The listing builds one solid part. Answer for the finished solid, in the listing's coordinates (mm). Round coordinates to 2 decimals unless told otherwise and drop trailing zeros. Order: outer loops, then holes, each group sorted by start corner. A loop starts at its lowest first (then second) coordinate and runs counter-clockwise, first axis right, second up. Notation, with made-up numbers: (13.25, 79) -> (50.25, 79) arc R30 cw to (50.25, 110) -> close; hole circle Ø6 at (-16, 64). An arc over 180 degrees is marked (long way). Answer in a Markdown table with one row per item. Add a question column.
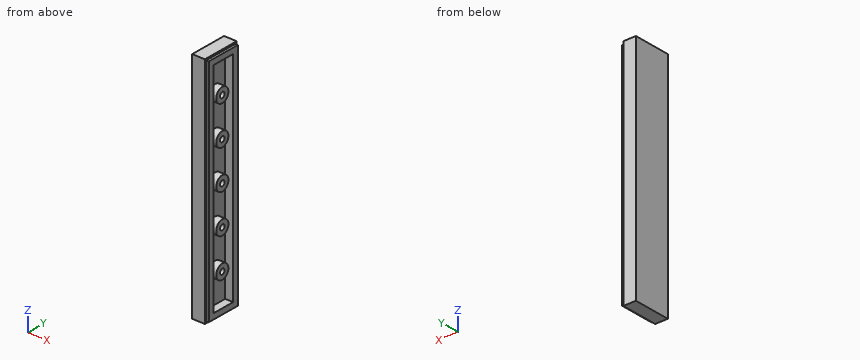
```python
from build123d import *

# Parameters (mm, degrees)
SKETCH1_W           = 47.79
SKETCH1_H           = 7.79
BOSS_EXTRUDE1_DEPTH = 2.63
SHELL1_T            = -1.5
SKETCH2_W           = 47.09
SKETCH2_H           = 7.09
SKETCH2_W_2         = 44.79
SKETCH2_H_2         = 4.79
BOSS_EXTRUDE2_DEPTH = 0.52
SKETCH3_R           = 1.485
SKETCH3_R_2         = 0.555
BOSS_EXTRUDE3_DEPTH = 1.45


with BuildPart() as part:
    # Sketch1 → Boss-Extrude1 (new body)
    with BuildSketch(Plane(origin=(0, 0, 0), x_dir=(0, 0, -1), z_dir=(1, 0, 0))):
        Rectangle(SKETCH1_W, SKETCH1_H)
    extrude(amount=BOSS_EXTRUDE1_DEPTH)

    # Shell1
    shell1_openings = [part.faces().sort_by_distance(p)[0] for p in [
        (2.63, 0, 0),
    ]]
    offset(amount=SHELL1_T, openings=shell1_openings, kind=Kind.INTERSECTION)

    # Sketch2 → Boss-Extrude2 (add)
    with BuildSketch(Plane(origin=(2.63, 0, 0), x_dir=(0, 0, -1), z_dir=(1, 0, 0))):
        Rectangle(SKETCH2_W, SKETCH2_H)
        Rectangle(SKETCH2_W_2, SKETCH2_H_2, mode=Mode.SUBTRACT)
    extrude(amount=BOSS_EXTRUDE2_DEPTH)

    # Sketch3 → Boss-Extrude3 (add)
    # profile 1 of 5: a face of its own
    with BuildSketch(Plane(origin=(1.5, 0, 0), x_dir=(0, 0, -1), z_dir=(1, 0, 0))):
        with Locations(Location((-15.93, 0, 0), (0, 0, 180))):
            Circle(SKETCH3_R)
        with Locations(Location((-15.93, 0, 0), (0, 0, 180))):
            Circle(SKETCH3_R_2, mode=Mode.SUBTRACT)
    # profile 2 of 5: a face of its own
    with BuildSketch(Plane(origin=(1.5, 0, 0), x_dir=(0, 0, -1), z_dir=(1, 0, 0))):
        with Locations(Location((-7.96, 0, 0), (0, 0, 180))):
            Circle(SKETCH3_R)
        with Locations(Location((-7.96, 0, 0), (0, 0, 180))):
            Circle(SKETCH3_R_2, mode=Mode.SUBTRACT)
    # profile 3 of 5: a face of its own
    with BuildSketch(Plane(origin=(1.5, 0, 0), x_dir=(0, 0, -1), z_dir=(1, 0, 0))):
        with Locations(Location((0.01, 0, 0), (0, 0, 180))):
            Circle(SKETCH3_R)
        with Locations(Location((0.01, 0, 0), (0, 0, 180))):
            Circle(SKETCH3_R_2, mode=Mode.SUBTRACT)
    # profile 4 of 5: a face of its own
    with BuildSketch(Plane(origin=(1.5, 0, 0), x_dir=(0, 0, -1), z_dir=(1, 0, 0))):
        with Locations(Location((7.98, 0, 0), (0, 0, 180))):
            Circle(SKETCH3_R)
        with Locations(Location((7.98, 0, 0), (0, 0, 180))):
            Circle(SKETCH3_R_2, mode=Mode.SUBTRACT)
    # profile 5 of 5: a face of its own
    with BuildSketch(Plane(origin=(1.5, 0, 0), x_dir=(0, 0, -1), z_dir=(1, 0, 0))):
        with Locations(Location((15.95, 0, 0), (0, 0, 180))):
            Circle(SKETCH3_R)
        with Locations(Location((15.95, 0, 0), (0, 0, 180))):
            Circle(SKETCH3_R_2, mode=Mode.SUBTRACT)
    extrude(amount=BOSS_EXTRUDE3_DEPTH)


solid = part.part
```
Item 1: The part is cut by section B-B, the plane z = 15.93. Give the vertices of the cut face in (x, y) (3 decimals), and give its area (3 significant figures).
Item 2: Find the intervals of material crossed by probe 1 along Y at (x, z) = (2.15, 7.96) (3 decimals); probe 2 along Y at (x, z) = (1.95, 1) (3 decimals); probe 3 along Z at (x, y) = (1.9, -1.75) (3 decimals), in increasing order. Write a range as [from, to].
Item 3: The part is cut by section C-C, the plane z = -16. Give the vertices of the cut face in (x, y) (3 decimals).
Item 4: The part is cut by section A-A, the plane z = -11. Give the vertices of the cut face in (x, y) (3 decimals).
Item 5: Flat-ended cylindrical pins translate along their axes: P1, Ø0.6, axis at x = 3, z = 4.5, coming from the -Y side (3 decimals); P2, Ø0.9, axis at y = 0, z = -16, coming from the +X side; P3, Ø0.9, axis at y = 0.5, z = 0.5, coming from the +X side. Find the tip coordinate at first contact, or state that the pin passes through.
Resolved:
| question | item | result |
|---|---|---|
| 1 | outline | (0, -3.895) -> (2.63, -3.895) -> (2.63, -3.545) -> (3.15, -3.545) -> (3.15, -2.395) -> (1.5, -2.395) -> (1.5, -1.485) -> (2.95, -1.485) -> (2.95, -0.555) -> (1.5, -0.555) -> (1.5, 0.555) -> (2.95, 0.555) -> (2.95, 1.485) -> (1.5, 1.485) -> (1.5, 2.395) -> (3.15, 2.395) -> (3.15, 3.545) -> (2.63, 3.545) -> (2.63, 3.895) -> (0, 3.895) -> close |
| 1 | area | 19.0 mm2 |
| 2 | probe 1 | [-3.895, -2.395], [-1.485, -0.555], [0.555, 1.485], [2.395, 3.895] |
| 2 | probe 2 | [-3.895, -2.395], [-1.089, 1.089], [2.395, 3.895] |
| 2 | probe 3 | [-23.895, -22.395], [22.395, 23.895] |
| 3 | outline | (0, -3.895) -> (2.63, -3.895) -> (2.63, -3.545) -> (3.15, -3.545) -> (3.15, -2.395) -> (1.5, -2.395) -> (1.5, -1.484) -> (2.95, -1.484) -> (2.95, -0.553) -> (1.5, -0.553) -> (1.5, 0.553) -> (2.95, 0.553) -> (2.95, 1.484) -> (1.5, 1.484) -> (1.5, 2.395) -> (3.15, 2.395) -> (3.15, 3.545) -> (2.63, 3.545) -> (2.63, 3.895) -> (0, 3.895) -> close |
| 4 | outline | (0, -3.895) -> (2.63, -3.895) -> (2.63, -3.545) -> (3.15, -3.545) -> (3.15, -2.395) -> (1.5, -2.395) -> (1.5, 2.395) -> (3.15, 2.395) -> (3.15, 3.545) -> (2.63, 3.545) -> (2.63, 3.895) -> (0, 3.895) -> close |
| 5 | P1 | y = -3.545 |
| 5 | P2 | x = 1.5 |
| 5 | P3 | x = 2.95 |
